```python
from build123d import *

# Parameters (mm, degrees)
F1_DEPTH = 1.5


# Not quite as in the source:
# - a feature names something its author has since deleted; it is built from what else it names


with BuildPart() as f1:
    # F0 (on Top) → F1 (new body)
    with BuildSketch(Plane.XY):
        with BuildLine():
            ThreePointArc((-4.7637764364, 4.2277344156), (-4.22987066, 3.4988615225), (-3.8857919263, 2.6634449214))
            Line((-3.8857919263, 2.6634449214), (1.5419516712, 3.0945423002))
            Line((1.5419516712, 3.0945423002), (-4.7637764364, 9))
            Line((-4.7637764364, 9), (-4.7637764364, 4.2277344156))
        make_face()
        with BuildLine():
            ThreePointArc((-7.5, -2.0865550786), (-6.0089576806, -1.7773824212), (-4.7637764364, -0.9008445729))
            Line((-4.7637764364, -0.9008445729), (-4.7637764364, 0.9063707553))
            Line((-4.7637764364, 0.9063707553), (-5.0905279509, 0.9967782547))
            ThreePointArc((-5.0905279509, 0.9967782547), (-5.986174823, -0.326111143), (-7.5, -0.8365550786))
            Line((-7.5, -0.8365550786), (-7.5, -2.0865550786))
        make_face()
        with BuildLine():
            Line((-4.7637764364, 2.4205190875), (-4.7637764364, 4.2277344156))
            ThreePointArc((-4.7637764364, 4.2277344156), (-6.0089576806, 5.104272264), (-7.5, 5.4134449214))
            Line((-7.5, 5.4134449214), (-7.5, 4.1634449214))
            ThreePointArc((-7.5, 4.1634449214), (-5.986174823, 3.6530009858), (-5.0905279509, 2.330111588))
            Line((-5.0905279509, 2.330111588), (-4.7637764364, 2.4205190875))
        make_face()
        with BuildLine():
            Line((-10.5388853699, 1.6634449214), (-10.5388853699, 3.8606421607))
            ThreePointArc((-10.5388853699, 3.8606421607), (-11.0677948468, 2.8181483168), (-11.25, 1.6634449214))
            Line((-11.25, 1.6634449214), (-10.5388853699, 1.6634449214))
        make_face()
        with BuildLine():
            ThreePointArc((-11.25, 1.6634449214), (-11.0677948468, 0.5087415259), (-10.5388853699, -0.533752318))
            Line((-10.5388853699, -0.533752318), (-10.5388853699, 1.6634449214))
            Line((-10.5388853699, 1.6634449214), (-11.25, 1.6634449214))
        make_face()
        with BuildLine():
            Line((1.5419516712, 0.2323475426), (-3.8857919263, 0.6634449214))
            ThreePointArc((-3.8857919263, 0.6634449214), (-4.22987066, -0.1719716798), (-4.7637764364, -0.9008445729))
            Line((-4.7637764364, -0.9008445729), (-4.7637764364, -5.4970695637))
            Line((-4.7637764364, -5.4970695637), (1.5419516712, 0.2323475426))
        make_face()
        with BuildLine():
            Line((-4.7637764364, -5.4970695637), (-4.7637764364, -0.9008445729))
            ThreePointArc((-4.7637764364, -0.9008445729), (-6.0089576806, -1.7773824212), (-7.5, -2.0865550786))
            ThreePointArc((-7.5, -2.0865550786), (-8.8586144698, -1.831789938), (-10.0326275495, -1.102110664))
            ThreePointArc((-10.0326275495, -1.102110664), (-10.300213716, -0.8308091044), (-10.5388853699, -0.533752318))
            Line((-10.5388853699, -0.533752318), (-10.5388853699, -5.4970695637))
            Line((-10.5388853699, -5.4970695637), (-4.7637764364, -5.4970695637))
        make_face()
        with BuildLine():
            ThreePointArc((-7.5, 5.4134449214), (-6.0089576806, 5.104272264), (-4.7637764364, 4.2277344156))
            Line((-4.7637764364, 4.2277344156), (-4.7637764364, 9))
            Line((-4.7637764364, 9), (-10.5388853699, 9))
            Line((-10.5388853699, 9), (-10.5388853699, 3.8606421607))
            ThreePointArc((-10.5388853699, 3.8606421607), (-10.2477408327, 4.2153893401), (-9.9154440374, 4.5319166577))
            ThreePointArc((-9.9154440374, 4.5319166577), (-8.7856381662, 5.1861760359), (-7.5, 5.4134449214))
        make_face()
        with BuildLine():
            Line((-10.5388853699, 3.8606421607), (-10.5388853699, 9))
            Line((-10.5388853699, 9), (-14.1904987395, 4.4458052143))
            Line((-14.1904987395, 4.4458052143), (-14.1904987395, -0.9716537897))
            Line((-14.1904987395, -0.9716537897), (-10.5388853699, -5.4970695637))
            Line((-10.5388853699, -5.4970695637), (-10.5388853699, -0.533752318))
            ThreePointArc((-10.5388853699, -0.533752318), (-11.0677948468, 0.5087415259), (-11.25, 1.6634449214))
            ThreePointArc((-11.25, 1.6634449214), (-11.0677948468, 2.8181483168), (-10.5388853699, 3.8606421607))
        make_face()
        with BuildLine():
            ThreePointArc((-4.7637764364, -0.9008445729), (-4.22987066, -0.1719716798), (-3.8857919263, 0.6634449214))
            Line((-3.8857919263, 0.6634449214), (-4.7637764364, 0.9063707553))
            Line((-4.7637764364, 0.9063707553), (-4.7637764364, -0.9008445729))
        make_face()
        with BuildLine():
            Line((-4.7637764364, 2.4205190875), (-3.8857919263, 2.6634449214))
            ThreePointArc((-3.8857919263, 2.6634449214), (-4.22987066, 3.4988615225), (-4.7637764364, 4.2277344156))
            Line((-4.7637764364, 4.2277344156), (-4.7637764364, 2.4205190875))
        make_face()
    extrude(amount=F1_DEPTH)


solid = f1.part
```
Geometry check sheet. Reference: the model listing, model coordinates, mm. A direction names the side the tool comes from. Round coordinates to 2 decimals unless told otherwise and drop trailing zeros. Loops run counter-clockwise (first coordinate to the right, second up) from the corner with the lowest first, then second, coordinate; pieces in that order, holes last. Notation, with made-up numbers: (6, -16) - (38, -16) arc R14 ccw to (38, 9) - close; hole circle Ø2 at (-37, -24.75). An arc over 180 degrees is marked (long way). Use a Markdown table: item, result.
Q1. Cross-section at C-C on z = 0.85. Record the cut outline in (x, y), plus the area to 3 significant figures.
Solutions:
| item | result |
|---|---|
| outline | (-14.19, -0.97) - (-10.54, -5.5) - (-4.76, -5.5) - (1.54, 0.23) - (-3.89, 0.66) - (-5.09, 1) arc R2.5 cw to (-7.5, -0.84) - (-7.5, -2.09) arc R3.75 cw to (-10.54, -0.53) - (-10.54, 3.86) arc R3.75 cw to (-7.5, 5.41) - (-7.5, 4.16) arc R2.5 cw to (-5.09, 2.33) - (-3.89, 2.66) - (1.54, 3.09) - (-4.76, 9) - (-10.54, 9) - (-14.19, 4.45) - close |
| area | 130 mm2 |
Q2. Cross-section at D-D on x = -12.25. Record the cut outline in (y, z).
Solutions:
| item | result |
|---|---|
| outline | (-3.38, 0) - (6.87, 0) - (6.87, 1.5) - (-3.38, 1.5) - close |
Q3. Access from +Z, -Z, +X, -X, +Y, -Y to the whole of each face (thin tool, end or side, straight path). Record for faces 4 (the flat face through (-8, -5.497, 1)), 5 (the flat face through (-1.21, 2.876, 0.74)), 6 (the cylindrical face through (-5.968, -0.312, 0.74)).
Solutions:
| item | result |
|---|---|
| face 4 | +Z, -Z, +X, -X, -Y |
| face 5 | +Z, -Z, +X |
| face 6 | +Z, -Z |
Q4. Cross-section at B-B on x = -6.5. Record the cut outline in (y, z), plus the area to 3 significant figures.
Solutions:
| item | result |
|---|---|
| outline | (-5.5, 0) - (-0.63, 0) - (-0.63, 1.5) - (-5.5, 1.5) - close; (3.95, 0) - (9, 0) - (9, 1.5) - (3.95, 1.5) - close |
| area | 14.9 mm2 |
Q5. Cross-section at A-A on y = 4.75. Record the cut outline in (x, z).
Solutions:
| item | result |
|---|---|
| outline | (-13.95, 0) - (-9.63, 0) - (-9.63, 1.5) - (-13.95, 1.5) - close; (-7.5, 0) - (-0.23, 0) - (-0.23, 1.5) - (-7.5, 1.5) - close |
Q6. Material ranges on line 1 (Y direction, x = 0.5, z = 1.15); line 2 (X direction, y = -0.5, z = 1.45); line 3 (X direction, y = 4.25, z = 0.4), recorded low to high.
Solutions:
| item | result |
|---|---|
| line 1 | y = -0.71 to 0.32, 3.01 to 4.07 |
| line 2 | x = -14.19 to -10.54, -6.25 to 0.74 |
| line 3 | x = -14.19 to -10.22, -7.5 to 0.31 |
Q7. Draft check along Y on faces 1 (the flat face through (-14.19, 2, 1)), 2 (the flat face through (-7.5, -1, 1)), 3 (the flat face through (-12.39, -3.2, 0.74)). Enter one of: released by +Y, released by -Y, zero draft, split by the parting line, or undercut.
Solutions:
| item | result |
|---|---|
| face 1 | zero draft |
| face 2 | undercut |
| face 3 | released by -Y |
